Here's how the part is built. I have some questions about the finished solid (model axes, mm). A direction names the side the tool comes from. Round coordinates to 2 decimals unless told otherwise and drop trailing zeros. Write each loop counter-clockwise with the first axis right and the second up, starting at its lowest first coordinate (ties: lowest second). Pieces come first, ordered by that corner, then holes. Notation, with made-up numbers: (5.5, -8.75) -> (36.5, -8.75) arc R21 ccw to (36.5, 26.25) -> close; hole circle Ø10 at (-20, 0). An arc over 180 degrees is marked (long way). Answer in a Markdown table with one row per item.
from build123d import *

# Parameters (mm, degrees)
F0_W     = 584.2
F0_H     = 219.71
F1_DEPTH = 5.334
F2_W     = 571.5
F2_H     = 213.36
F2_W_2   = 546.1
F2_H_2   = 187.96
F3_DEPTH = 12.7
F4_R     = 25.4
F6_DEPTH = 12.7
F7_W     = 12.7
F7_H     = 109.855
F8_DEPTH = 5.334


# Not quite as in the source:
# - a feature names something its author has since deleted; it is built from what else it names


with BuildPart() as f1:
    # F0 (on Front) → F1 (new body)
    with BuildSketch(Plane.XZ):
        with Locations((-292.1, 109.855)):
            Rectangle(F0_W, F0_H)
    extrude(amount=F1_DEPTH)

    # F2 (on face) → F3 (join)
    with BuildSketch(Plane.XZ.offset(5.334)):
        with Locations((-292.1, 113.03)):
            Rectangle(F2_W, F2_H)
        with Locations((-292.1, 113.03)):
            Rectangle(F2_W_2, F2_H_2, mode=Mode.SUBTRACT)
    extrude(amount=F3_DEPTH)

    # F4
    f4_edges = [f1.edges().sort_by_distance(p)[0] for p in [
        (-565.15, -11.684, 207.01),
        (-19.05, -11.684, 207.01),
        (-19.05, -11.684, 19.05),
        (-565.15, -11.684, 19.05),
    ]]
    fillet(f4_edges, radius=F4_R)

    # F5 (on face) → F6 (cut)
    with BuildSketch(Plane.XZ.offset(18.034)):
        Polygon((-118.11, 219.71), (-125.73, 207.01), (-118.11, 207.01), (-113.5820166854, 214.5566388576), (-110.49, 219.71), align=None)
        Polygon((-56.5979833146, 214.5566388576), (-52.07, 207.01), (-44.45, 207.01), (-52.07, 219.71), (-59.69, 219.71), align=None)
        Polygon((-59.69, 219.71), (-110.49, 219.71), (-113.5820166854, 214.5566388576), (-56.5979833146, 214.5566388576), align=None)
    extrude(amount=-F6_DEPTH, mode=Mode.SUBTRACT)

    # F7 (on face) → F8 (join)
    with BuildSketch(Plane(origin=(0, 0, 0), x_dir=(-1, 0, 0), z_dir=(0, 1, 0))):
        with BuildLine():
            Line((292.1, 0), (0, 0))
            Line((0, 0), (-12.7, 0))
            Line((-12.7, 0), (-12.7, -18.4187279276))
            Line((-12.7, -18.4187279276), (273.05, -18.4187279276))
            add(Edge.make_bspline(
                [(292.1, 0), (287.6007994264, -5.2493532032), (283.1015988528, -10.4987064064), (273.05, -18.4187279276)],
                knots=[0, 0, 0, 0, 0.0728769887, 0.0728769887, 0.0728769887, 0.0728769887], degree=3))
        make_face()
        with Locations((-6.35, 54.9275)):
            Rectangle(F7_W, F7_H)
        with BuildLine():
            Line((-12.7, -18.4187279276), (-12.7, 0))
            Line((-12.7, 0), (-12.7, 109.855))
            Line((-12.7, 109.855), (-44.45, 109.855))
            add(Edge.make_bspline(
                [(-45.0211916342, 91.2168765815), (-45.0211916609, 97.5162300277), (-44.815953395, 103.7471754572), (-44.45, 109.855)],
                knots=[0.5639304479, 0.5639304479, 0.5639304479, 0.5639304479, 0.5870347541, 0.5870347541, 0.5870347541, 0.5870347541], degree=3))
            add(Edge.make_bspline(
                [(-12.7, -18.4187279276), (-37.5240442459, 12.5724048939), (-45.0211914731, 53.1440785365), (-45.0211916342, 91.2168765815)],
                knots=[0.4242898339, 0.4242898339, 0.4242898339, 0.4242898339, 0.5639304479, 0.5639304479, 0.5639304479, 0.5639304479], degree=3))
        make_face()
        with BuildLine():
            Line((584.2, 0), (292.1, 0))
            add(Edge.make_bspline(
                [(292.1, 0), (296.5992005736, -5.2493532032), (301.0984011472, -10.4987064064), (311.15, -18.4187279276)],
                knots=[0, 0, 0, 0, 0.0728769887, 0.0728769887, 0.0728769887, 0.0728769887], degree=3))
            Line((311.15, -18.4187279276), (596.9, -18.4187279276))
            Line((596.9, -18.4187279276), (596.9, 0))
            Line((596.9, 0), (584.2, 0))
        make_face()
        with BuildLine():
            Line((-12.7, 109.855), (0, 109.855))
            Line((0, 109.855), (0, 219.71))
            add(Edge.make_bspline(
                [(-12.7, 204.8965850641), (-8.9139816017, 209.8723459181), (-4.696536047, 214.8060326557), (0, 219.71)],
                knots=[0.7188244338, 0.7188244338, 0.7188244338, 0.7188244338, 0.7411532433, 0.7411532433, 0.7411532433, 0.7411532433], degree=3))
            Line((-12.7, 204.8965850641), (-12.7, 109.855))
        make_face()
        with BuildLine():
            Line((-44.45, 109.855), (-12.7, 109.855))
            Line((-12.7, 109.855), (-12.7, 204.8965850641))
            add(Edge.make_bspline(
                [(-44.45, 109.855), (-42.3625587956, 144.6947495266), (-35.0459362357, 175.5285199707), (-12.7, 204.8965850641)],
                knots=[0.5870347541, 0.5870347541, 0.5870347541, 0.5870347541, 0.7188244338, 0.7188244338, 0.7188244338, 0.7188244338], degree=3))
        make_face()
        with BuildLine():
            Line((273.05, -18.4187279276), (-12.7, -18.4187279276))
            add(Edge.make_bspline(
                [(101.1778231225, -76.2), (55.3698473988, -71.3735043498), (12.4455878923, -49.8112861475), (-12.7, -18.4187279276)],
                knots=[0.2828404673, 0.2828404673, 0.2828404673, 0.2828404673, 0.4242898339, 0.4242898339, 0.4242898339, 0.4242898339], degree=3))
            Line((101.1778231225, -76.2), (139.7, -76.2))
            add(Edge.make_bspline(
                [(273.05, -18.4187279276), (249.5100545477, -36.9667099273), (195.5177305995, -70.1620926298), (139.7, -76.2)],
                knots=[0.0728769887, 0.0728769887, 0.0728769887, 0.0728769887, 0.2435483779, 0.2435483779, 0.2435483779, 0.2435483779], degree=3))
        make_face()
        with BuildLine():
            Line((596.9, -18.4187279276), (311.15, -18.4187279276))
            add(Edge.make_bspline(
                [(311.15, -18.4187279276), (334.6899454523, -36.9667099273), (388.6822694005, -70.1620926298), (444.5, -76.2)],
                knots=[0.0728769887, 0.0728769887, 0.0728769887, 0.0728769887, 0.2435483779, 0.2435483779, 0.2435483779, 0.2435483779], degree=3))
            Line((444.5, -76.2), (483.0221768775, -76.2))
            add(Edge.make_bspline(
                [(483.0221768775, -76.2), (528.8301526012, -71.3735043498), (571.7544121077, -49.8112861475), (596.9, -18.4187279276)],
                knots=[0.2828404673, 0.2828404673, 0.2828404673, 0.2828404673, 0.4242898339, 0.4242898339, 0.4242898339, 0.4242898339], degree=3))
        make_face()
        with Locations((590.55, 54.9275)):
            Rectangle(F7_W, F7_H)
        with BuildLine():
            add(Edge.make_bspline(
                [(0, 219.71), (3.0172855437, 222.8605496023), (6.2323113272, 225.9988327955), (9.6341187106, 229.1255293763)],
                knots=[0.7411532433, 0.7411532433, 0.7411532433, 0.7411532433, 0.7554983677, 0.7554983677, 0.7554983677, 0.7554983677], degree=3))
            Line((0, 219.71), (292.1, 219.71))
            Line((292.1, 219.71), (9.6341187106, 229.1255293763))
        make_face()
        with BuildLine():
            Line((596.9, 0), (596.9, -18.4187279276))
            add(Edge.make_bspline(
                [(596.9, -18.4187279276), (621.7240438178, 12.5724043593), (629.2211912145, 53.144077137), (629.2211916342, 91.2168746116)],
                knots=[0.4242898339, 0.4242898339, 0.4242898339, 0.4242898339, 0.5639304455, 0.5639304455, 0.5639304455, 0.5639304455], degree=3))
            add(Edge.make_bspline(
                [(629.2211916342, 91.2168746116), (629.2211917037, 97.5162287286), (629.0159534331, 103.7471748205), (628.65, 109.855)],
                knots=[0.5639304455, 0.5639304455, 0.5639304455, 0.5639304455, 0.5870347541, 0.5870347541, 0.5870347541, 0.5870347541], degree=3))
            Line((628.65, 109.855), (596.9, 109.855))
            Line((596.9, 109.855), (596.9, 0))
        make_face()
        with BuildLine():
            Line((584.2, 219.71), (584.2, 109.855))
            Line((584.2, 109.855), (596.9, 109.855))
            Line((596.9, 109.855), (596.9, 204.8965850641))
            add(Edge.make_bspline(
                [(596.9, 204.8965850641), (593.1139816017, 209.8723459181), (588.896536047, 214.8060326557), (584.2, 219.71)],
                knots=[0.7188244338, 0.7188244338, 0.7188244338, 0.7188244338, 0.7411532433, 0.7411532433, 0.7411532433, 0.7411532433], degree=3))
        make_face()
        with BuildLine():
            add(Edge.make_bspline(
                [(9.6341187106, 229.1255293763), (9.9041896656, 229.3737591661), (10.1754378752, 229.6219159272), (10.4478578559, 229.87)],
                knots=[0.7554983677, 0.7554983677, 0.7554983677, 0.7554983677, 0.7566372333, 0.7566372333, 0.7566372333, 0.7566372333], degree=3))
            Line((9.6341187106, 229.1255293763), (292.1, 219.71))
            Line((292.1, 219.71), (574.5658812894, 229.1255293763))
            add(Edge.make_bspline(
                [(574.5658812894, 229.1255293763), (574.2958103344, 229.3737591661), (574.0245621248, 229.6219159272), (573.7521421441, 229.87)],
                knots=[0.7554983677, 0.7554983677, 0.7554983677, 0.7554983677, 0.7566372333, 0.7566372333, 0.7566372333, 0.7566372333], degree=3))
            Line((573.7521421441, 229.87), (514.35, 229.87))
            Line((514.35, 229.87), (292.1, 229.87))
            Line((292.1, 229.87), (69.85, 229.87))
            Line((69.85, 229.87), (10.4478578559, 229.87))
        make_face()
        with BuildLine():
            Line((574.5658812894, 229.1255293763), (292.1, 219.71))
            Line((292.1, 219.71), (584.2, 219.71))
            add(Edge.make_bspline(
                [(584.2, 219.71), (581.1827144563, 222.8605496023), (577.9676886728, 225.9988327955), (574.5658812894, 229.1255293763)],
                knots=[0.7411532433, 0.7411532433, 0.7411532433, 0.7411532433, 0.7554983677, 0.7554983677, 0.7554983677, 0.7554983677], degree=3))
        make_face()
        with BuildLine():
            Line((596.9, 204.8965850641), (596.9, 109.855))
            Line((596.9, 109.855), (628.65, 109.855))
            add(Edge.make_bspline(
                [(628.65, 109.855), (626.5625587956, 144.6947495266), (619.2459362357, 175.5285199707), (596.9, 204.8965850641)],
                knots=[0.5870347541, 0.5870347541, 0.5870347541, 0.5870347541, 0.7188244338, 0.7188244338, 0.7188244338, 0.7188244338], degree=3))
        make_face()
        with BuildLine():
            add(Edge.make_bspline(
                [(10.4478578559, 229.87), (68.6609423687, 282.8827748158), (180.3804711844, 332.5763874079), (292.1, 382.27)],
                knots=[0.7566372333, 0.7566372333, 0.7566372333, 0.7566372333, 1, 1, 1, 1], degree=3))
            Line((10.4478578559, 229.87), (69.85, 229.87))
            Line((69.85, 229.87), (292.1, 229.87))
            Line((292.1, 229.87), (292.1, 382.27))
        make_face()
        with BuildLine():
            add(Edge.make_bspline(
                [(573.7521421441, 229.87), (515.5390576313, 282.8827748158), (403.8195288156, 332.5763874079), (292.1, 382.27)],
                knots=[0.7566372333, 0.7566372333, 0.7566372333, 0.7566372333, 1, 1, 1, 1], degree=3))
            Line((292.1, 382.27), (292.1, 229.87))
            Line((292.1, 229.87), (514.35, 229.87))
            Line((514.35, 229.87), (573.7521421441, 229.87))
        make_face()
    extrude(amount=-F8_DEPTH)


solid = f1.part
1) For pin 1 (4 mm diameter, centred on y = -9.5, z = 108.5, fed in from +X); pin 2 (6.5 mm diameter, centred on x = -249, y = -9.5, fed in from -Z); pin 3 (10 mm diameter, centred on x = -340.5, y = -6, fed in from +Z), each with a flat end and sliding along its axis, tell me the tip position at first contact or that it passes through.
Response:
| item | result |
|---|---|
| pin 1 | stops at x = -6.35 |
| pin 2 | stops at z = 6.35 |
| pin 3 | stops at z = 362.89 |
2) We'd pull the mould along Z, two halves only. Please class faces 5 (the face through (-6.35, -12, 112)), 6 (the face through (-86, -12, 207.01)), 7 (the face through (-85, -12, 214.557)): +Z half, -Z half, draft (parallel to the pull), parting line (faces both ways), or undercut.
Response:
| item | result |
|---|---|
| face 5 | draft |
| face 6 | undercut |
| face 7 | +Z half |
3) Which directions (+Z, -Z, +X, -X, +Y, -Y) give clear straight access to the entire face, cutting with the end or side of a thin tool? Please do faces 1 (the face through (-577.85, -12, 112)), 2 (the face through (-351, -12, 219.71)), 3 (the face through (-121.867, -11.773, 213.449)), 4 (the face through (-296, -12, 6.35)).
Response:
| item | result |
|---|---|
| face 1 | +Z, -Z, -X, -Y |
| face 2 | +Z, +X, -X, -Y |
| face 3 | -Y |
| face 4 | -Z, +X, -X, -Y |
4) I need wall thicknesses on line 1 (Z direction, x = -172.5, y = -8); line 2 (Z direction, x = -103, y = -17); line 3 (X direction, y = -13, z = 219.5). Which ranges of each line are inside material? Lowest first, please. Write a range as [from, to].
Response:
| item | result |
|---|---|
| line 1 | z = [6.35, 19.05], [207.01, 219.71] |
| line 2 | z = [6.35, 19.05], [207.01, 214.56] |
| line 3 | x = [-577.85, -118.24], [-51.94, -6.35] |
5) I want a section at A-A, the plane y = -13.25. List the corners of the cut face in (x, z) for me.
Response:
| item | result |
|---|---|
| outline | (-577.85, 6.35) -> (-6.35, 6.35) -> (-6.35, 219.71) -> (-52.07, 219.71) -> (-44.45, 207.01) arc R25.4 cw to (-19.05, 181.61) -> (-19.05, 44.45) arc R25.4 cw to (-44.45, 19.05) -> (-539.75, 19.05) arc R25.4 cw to (-565.15, 44.45) -> (-565.15, 181.61) arc R25.4 cw to (-539.75, 207.01) -> (-125.73, 207.01) -> (-118.11, 219.71) -> (-577.85, 219.71) -> close; (-118.11, 207.01) -> (-52.07, 207.01) -> (-56.6, 214.56) -> (-113.58, 214.56) -> close |
